Build history of the part. All positions in model axes, mm. Face numbers are marked on the shaded views. A direction names the side the tool comes from. Round coordinates to 2 decimals unless told otherwise and drop trailing zeros. Write each loop counter-clockwise with the first axis right and the second up, starting at its lowest first coordinate (ties: lowest second). Pieces come first, ordered by that corner, then holes. Notation, with made-up numbers: M -21.75,59 L 11.25,59 A21 cw 11.25,69 Z; hole C 23.25,-10.75 d9. An arc over 180 degrees is marked long. Write item = value, one per line.
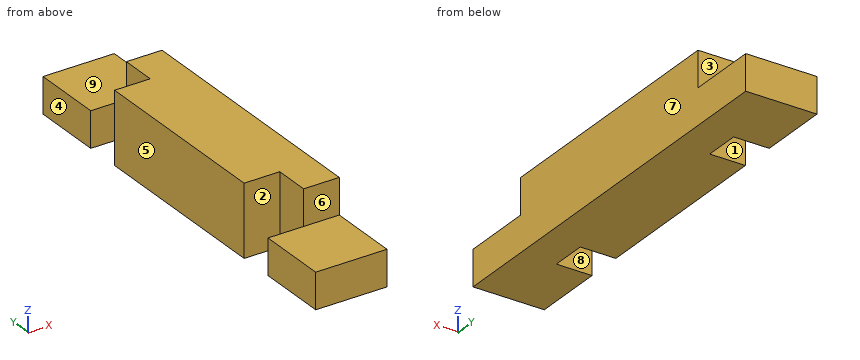
from build123d import *

# Parameters (mm, degrees)
F0_W     = 44.45
F0_H     = 44.45
F1_DEPTH = 254
F2_W     = 44.45
F2_H     = 44.45
F3_DEPTH = 22.225
F4_W     = 22.225
F4_H     = 44.45
F5_DEPTH = 22.225


with BuildPart() as f1:
    # F0 (on Front) → F1 (new body)
    with BuildSketch(Plane.XZ):
        with Locations((22.225, 22.225)):
            Rectangle(F0_W, F0_H)
    extrude(amount=F1_DEPTH)

    # F2 (on face) → F3 (cut)
    with BuildSketch(Plane.XY.offset(44.45)):
        with Locations((22.225, -231.775)):
            Rectangle(F2_W, F2_H)
        with Locations((22.225, -22.225)):
            Rectangle(F2_W, F2_H)
    extrude(amount=-F3_DEPTH, mode=Mode.SUBTRACT)

    # F4 (on face) → F5 (cut)
    with BuildSketch(Plane(origin=(0, 0, 0), x_dir=(0, -1, 0), z_dir=(-1, 0, 0))):
        with Locations((55.5625, 22.225)):
            Rectangle(F4_W, F4_H)
        with Locations((198.4375, 22.225)):
            Rectangle(F4_W, F4_H)
    extrude(amount=-F5_DEPTH, mode=Mode.SUBTRACT)


solid = f1.part
1. Mould opens along Y. For the marked faces 1, 2, 3 and 4 say: pulls with the +Y half, pulls with the -Y half, needs draft (parallel to the pull), parting line crosses it, or undercut.
Responses:
face_1 = undercut
face_2 = undercut
face_3 = pulls with the +Y half
face_4 = needs draft
2. Band-saw the part on B-B (z = 18). List the corners of the cut face in (x, y) (3 decimals).
Responses:
outline = M 0,-254 L 44.45,-254 L 44.45,0 L 0,0 L 0,-44.45 L 22.225,-44.45 L 22.225,-66.675 L 0,-66.675 L 0,-187.325 L 22.225,-187.325 L 22.225,-209.55 L 0,-209.55 Z
3. Band-saw the part on C-C (x = 35). List the corners of the cut face in (y, z) (3 decimals).
Responses:
outline = M -254,0 L 0,0 L 0,22.225 L -44.45,22.225 L -44.45,44.45 L -209.55,44.45 L -209.55,22.225 L -254,22.225 Z
4. Probe probe 1 along Y at (x, z) = (19, 16) (3 decimals); probe 2 along Y at (x, z) = (41.5, 23.5); probe 3 along Y at (x, z) = (18.5, 37.5) (3 decimals). List the from-to ranges inside material, lowest first.
Responses:
probe_1 = -254 to -209.55, -187.325 to -66.675, -44.45 to 0
probe_2 = -209.55 to -44.45
probe_3 = -187.325 to -66.675
5. Band-saw the part on D-D (z = 38.5). List the corners of the cut face in (x, y) (3 decimals).
Responses:
outline = M 0,-187.325 L 22.225,-187.325 L 22.225,-209.55 L 44.45,-209.55 L 44.45,-44.45 L 22.225,-44.45 L 22.225,-66.675 L 0,-66.675 Z
6. Flat gauge pins, fed straight in: pin 1 (5 mm diameter, centred on x = 21, z = 39, fed in from +Y); pin 2 (2 mm diameter, centred on x = 5, y = -39.5, fed in from +Z) (3 decimals); pin 3 (6.5 mm diameter, centred on x = 13, z = 28.5, fed in from -Y) (3 decimals). Where does each tip first touch, or does it go through?
Responses:
pin_1 = -44.45
pin_2 = 22.225
pin_3 = -187.325
7. Tool access for the marked faces 5, 6, 7, 8 and 9: list every direction of +Z, -Z, +X, -X, +Y, -Y with a clear straight run to the whole face (end or side of a thin tool).
Responses:
face_5 = +Z, -Z, -X, +Y, -Y
face_6 = +Z, +X, -X, -Y
face_7 = +Z, -Z, +X, +Y, -Y
face_8 = +Z, -Z, -X
face_9 = +Z, +X, -X, +Y
8. Band-saw the part on A-A (x = 20). List the corners of the cut face in (y, z) (3 decimals).
Responses:
outline = M -254,0 L -209.55,0 L -209.55,22.225 L -254,22.225 Z; M -187.325,0 L -66.675,0 L -66.675,44.45 L -187.325,44.45 Z; M -44.45,0 L 0,0 L 0,22.225 L -44.45,22.225 Z
